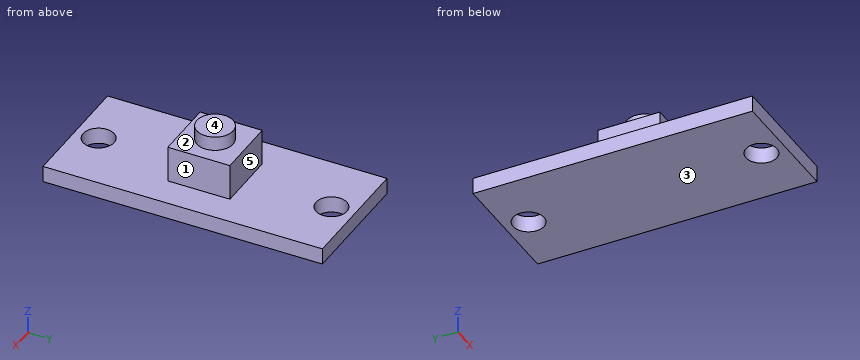
```python
from build123d import *

# Parameters (mm, degrees)
SKETCH1_W               = 12.192
SKETCH1_H               = 27.432
BOSS_EXTRUDE1_DEPTH     = 1.6002
SKETCH2_W               = 6.096
SKETCH2_H               = 6.096
BOSS_EXTRUDE2_DEPTH     = 3.556
CUT_EXTRUDE1_DEPTH      = 16.425142074
CUT_EXTRUDE1_DEPTH_BACK = 16.425142074
SKETCH4_R               = 1.524
SKETCH5_R               = 1.778
BOSS_EXTRUDE3_DEPTH     = 1.39954


with BuildPart() as part:
    # Sketch1 → Boss-Extrude1 (new body)
    with BuildSketch(Plane.XY):
        Rectangle(SKETCH1_W, SKETCH1_H)
    extrude(amount=BOSS_EXTRUDE1_DEPTH)

    # Sketch2 → Boss-Extrude2 (add)
    with BuildSketch(Plane.XY.offset(1.6002)):
        Rectangle(SKETCH2_W, SKETCH2_H)
    extrude(amount=BOSS_EXTRUDE2_DEPTH)

    # Sketch4 → Cut-Extrude1 (cut, two sides: drawn at the far end of the back side and taken through both)
    with BuildSketch(Plane.XY.offset(1.6002).offset(-CUT_EXTRUDE1_DEPTH_BACK)):
        with Locations((0, 11.43)):
            Circle(SKETCH4_R)
        with Locations((0, -11.43)):
            Circle(SKETCH4_R)
    extrude(amount=CUT_EXTRUDE1_DEPTH + CUT_EXTRUDE1_DEPTH_BACK, mode=Mode.SUBTRACT)

    # Sketch5 → Boss-Extrude3 (add)
    with BuildSketch(Plane.XY.offset(5.1562)):
        Circle(SKETCH5_R)
    extrude(amount=BOSS_EXTRUDE3_DEPTH)


solid = part.part
```
Model file for the job. Use its own axes, mm. Face numbers are marked on the shaded views. A direction names the side the tool comes from. Give positions to 0.01 mm unless a question says otherwise; leave off trailing zeros. Write each loop counter-clockwise with the first axis right and the second up, starting at its lowest first coordinate (ties: lowest second). Pieces come first, ordered by that corner, then holes. Notation, with made-up numbers: (27, -36.75) - (33, -36.75) arc R20 cw to (33, -1.75) - close; hole circle Ø1 at (-18, 22.5). An arc over 180 degrees is marked (long way). One line per question, with ' | ' between items. Start each with the question number.
(1) 3-axis set-ups, long thin cutter, end or side, ignore diameter. For the marked faces 1, 2, 3, 4 and 5: which of +Z, -Z, +X, -X, +Y, -Y reach the whole face in a straight line?
(2) Slice it at C-C on y = 0. Write the cut outline in (x, z), plus the area to 3 significant figures.
(3) Wall check: line 1 along Y through (x, z) = (0, 0.8); line 2 along X through (y, z) = (-11.43, 0.8); line 3 along Y through (x, z) = (-0.75, 0.5). Give the ranges that are in metal, low to high. Write a range as from..to.
(4) Slice it at D-D on z = 0.5. Write the cut outline in (x, y).
(5) Pin check, flat tips, straight feed: P1, Ø3.5, axis at x = 0, y = 11.43, coming from the -Z side; P2, Ø1.1, axis at x = 0.5, z = 3, coming from the +Y side; P3, Ø1.8, axis at y = -0.5, z = 3, coming from the +X side; P4, Ø2.5, axis at x = 0, y = -11.43, coming from the +Z side. Stop position of each tip, or through.
(6) Slice it at A-A on y = 11.43. Write the cut outline in (x, z), plus the area to 3 significant figures.
(7) Slice it at B-B on x = 0. Write the cut outline in (y, z).
Results below:
1) face 1: +Z, +X, +Y, -Y | face 2: +Z | face 3: -Z, +X, -X, +Y, -Y | face 4: +Z, +X, -X, +Y, -Y | face 5: +Z, +X, -X, +Y
2) outline: (-6.1, 0) - (6.1, 0) - (6.1, 1.6) - (3.05, 1.6) - (3.05, 5.16) - (1.78, 5.16) - (1.78, 6.56) - (-1.78, 6.56) - (-1.78, 5.16) - (-3.05, 5.16) - (-3.05, 1.6) - (-6.1, 1.6) - close | area: 46.2 mm^2
3) line 1: -13.72..-12.95, -9.91..9.91, 12.95..13.72 | line 2: -6.1..-1.52, 1.52..6.1 | line 3: -13.72..-12.76, -10.1..10.1, 12.76..13.72
4) outline: (-6.1, -13.72) - (6.1, -13.72) - (6.1, 13.72) - (-6.1, 13.72) - close; hole circle Ø3.05 at (0, -11.43); hole circle Ø3.05 at (0, 11.43)
5) P1: z = 0 | P2: y = 3.05 | P3: x = 3.05 | P4: through
6) outline: (-6.1, 0) - (-1.52, 0) - (-1.52, 1.6) - (-6.1, 1.6) - close; (1.52, 0) - (6.1, 0) - (6.1, 1.6) - (1.52, 1.6) - close | area: 14.6 mm^2
7) outline: (-13.72, 0) - (-12.95, 0) - (-12.95, 1.6) - (-13.72, 1.6) - close; (-9.91, 0) - (9.91, 0) - (9.91, 1.6) - (3.05, 1.6) - (3.05, 5.16) - (1.78, 5.16) - (1.78, 6.56) - (-1.78, 6.56) - (-1.78, 5.16) - (-3.05, 5.16) - (-3.05, 1.6) - (-9.91, 1.6) - close; (12.95, 0) - (13.72, 0) - (13.72, 1.6) - (12.95, 1.6) - close
